Could you check a few things on this model? Use its own coordinates, in mm. A direction names the side the tool comes from. Give positions to 0.01 mm unless a question says otherwise; leave off trailing zeros. Loops run counter-clockwise (first coordinate to the right, second up) from the corner with the lowest first, then second, coordinate; pieces in that order, holes last. Notation, with made-up numbers: M 22,11.5 L 47,11.5 A23 ccw 47,36.5 Z; hole C 64,4.25 d9. An arc over 180 degrees is marked long. Return JSON: item names as keys, results as strings. Group by question number.
1. For faces 4 (the flat face through (-0.952, 45, 0)), 5 (the flat face through (0, 1.058, 3)), 6 (the flat face through (0, 47.058, 0)), 7 (the flat face through (-3, 38.646, -1)), which set-ups out of +Z, -Z, +X, -X, +Y, -Y let a thin tool reach every point of the face, with its end or its side?
2. If we section it at A-A (y = 34): Write out the boundary of the cut face in (x, z), plus the area to 3 significant figures.
3. Please list where these lines run through material, in increasing order: line 1 (X direction, y = 37, z = -0.5); line 2 (Y direction, x = 0.75, z = -7); line 3 (X direction, y = 30, z = 0.5).
4. If we mould it in two halves opening along Z, with no side actions, what happens to faces 1 (the conical face through (5.39, 24.66, 0.08)), 2 (the flat face through (0, 0, 0)), 3 (the cylindrical face through (-7.62, 11.1, -2.4))? For each: +Z half, -Z half, draft (parallel to the pull), parting line (faces both ways), or undercut.
5. If we section it at B-B (y = 5): Write out the boundary of the cut face in (x, z).
6. For pin 1 (1.2 mm diameter, centred on y = 43.5, z = 0.5, fed in from -X); pin 2 (1.8 mm diameter, centred on x = -5.5, z = 0, fed in from -Y); pin 3 (8 mm diameter, centred on y = 10.5, z = 5.5, fed in from +X), each with a flat end and sliding along its axis, tell me the tip position at first contact or that it passes through.
```python
from build123d import *

# Parameters (mm, degrees)
M2X0_4_TAPPED_HOLE1_D           = 1.6
M2X0_4_TAPPED_HOLE1_DEPTH       = 12.0000014
M2X0_4_TAPPED_HOLE1_CSINK_D     = 2.05
M2X0_4_TAPPED_HOLE1_CSINK_ANGLE = 90
M2X0_4_TAPPED_HOLE1_TIP         = 0.480688495
CUT_EXTRUDE1_DEPTH              = 5.0165


with BuildPart() as part:
    # Sketch2 → Revolve1 (revolve)
    with BuildSketch(Plane.XY, mode=Mode.PRIVATE) as revolve1_sk:
        with BuildLine():
            Line((0, 0), (2.713042009, 0))
            Line((2.713042009, 0), (2.713042009, 1.057855461))
            Line((2.713042009, 1.057855461), (7.9883, 1.057855461))
            Line((7.9883, 1.057855461), (7.9883, 20.863496467))
            ThreePointArc((7.9883, 20.863496467), (7.937074629, 20.995273421), (7.810296505, 21.057855461))
            ThreePointArc((7.810296505, 21.057855461), (7.9405339, 21.185977007), (7.9883, 21.362315629))
            Line((7.9883, 21.362315629), (7.9883, 37.057855461))
            Line((7.9883, 37.057855461), (3.4163, 37.057855461))
            Line((3.4163, 37.057855461), (3.4163, 38.64639819))
            Line((3.4163, 38.64639819), (2.924863894, 38.64639819))
            Line((2.924863894, 38.64639819), (2.924863894, 38.982086399))
            Line((2.924863894, 38.982086399), (1.888599244, 38.982086399))
            Line((1.888599244, 38.982086399), (1.888599244, 39.34639819))
            Line((1.888599244, 39.34639819), (1.5, 39.34639819))
            Line((1.5, 39.34639819), (1.5, 47.057855461))
            Line((1.5, 47.057855461), (0, 47.057855461))
            Line((0, 47.057855461), (0, 0))
        make_face()
    revolve(revolve1_sk.sketch.rotate(Axis((0, 47.057855461, 0), (0, -1, 0)), 180), axis=Axis((0, 47.057855461, 0), (0, -1, 0)))

    # M2x0.4 Tapped Hole1
    with Locations(Plane(origin=(0, 37.057855461, 0), x_dir=(1, 0, 0), z_dir=(0, 1, 0))):
        with Locations((-5.5, 0), (5.5, 0)):
            CounterSinkHole(M2X0_4_TAPPED_HOLE1_D / 2, M2X0_4_TAPPED_HOLE1_CSINK_D / 2, depth=M2X0_4_TAPPED_HOLE1_DEPTH, counter_sink_angle=M2X0_4_TAPPED_HOLE1_CSINK_ANGLE)
            with Locations((0, 0, -(M2X0_4_TAPPED_HOLE1_DEPTH + M2X0_4_TAPPED_HOLE1_TIP / 2))):  # 118° drill point
                Cone(0, M2X0_4_TAPPED_HOLE1_D / 2, M2X0_4_TAPPED_HOLE1_TIP, mode=Mode.SUBTRACT)

    # Sketch6 → Cut-Extrude1 (cut)
    with BuildSketch(Plane(origin=(0, 47.057855461, 0), x_dir=(1, 0, 0), z_dir=(0, 1, 0))):
        Polygon((-0.9525, -36.740540228), (-0.9525, -1.158768204), (-0.9525, 1.158768204), (-0.9525, 36.740540228), (-72.116044049, 36.740540228), (-72.116044049, -36.740540228), align=None)
    extrude(amount=-CUT_EXTRUDE1_DEPTH, mode=Mode.SUBTRACT)


solid = part.part
```
Answer:
{
 "1": {"face 4": "+Z, -Z, -X, +Y", "face 5": "-Y", "face 6": "+Z, -Z, +X, -X, +Y", "face 7": "+Y"},
 "2": {"outline": "C 0,0 d15.98; hole C -5.5,0 d1.6; hole C 5.5,0 d1.6", "area": "196 mm²"},
 "3": {"line 1": "x = -7.97 to -6.33, -4.67 to 4.67, 6.33 to 7.97", "line 2": "y = 1.06 to 37.06", "line 3": "x = -7.97 to -6.12, -4.88 to 4.88, 6.12 to 7.97"},
 "4": {"face 1": "undercut", "face 2": "draft", "face 3": "parting line"},
 "5": {"outline": "C 0,0 d15.98"},
 "6": {"pin 1": "stops at x = -0.95", "pin 2": "stops at y = 1.06", "pin 3": "stops at x = 7.85"}
}
